For this review, take the finished solid that the model builds, in its own axes (mm). Round coordinates to 2 decimals unless told otherwise and drop trailing zeros. Loops run counter-clockwise (first coordinate to the right, second up) from the corner with the lowest first, then second, coordinate; pieces in that order, holes last.
1) Take a section at B-B (x = 16). State the section outline as (y, z) points.
2) Wall thickness on L1, parallel to Z at x = 0, y = -279.5; L2, parallel to X at y = -57, z = 16; L3, parallel to X at y = -152, z = -17: over which ranges is each line inside the solid? List them lowest first.
3) Insertion check: pin 1 (1 mm diameter, centred on y = -84.5, z = -2.5, fed in from -X); pin 2 (10 mm diameter, centred on x = 0, y = -194, fed in from -Z) (3 decimals); pin 3 (2 mm diameter, centred on x = 3, y = -97.5, fed in from +Z). Each pin has a flat end and moves straight along its axis. Give the tip position at first contact, or say it passes through.
4) Take a section at A-A (z = 17). State the section outline as (x, y) points, then the cut area to 3 significant figures.
5) Take a section at C-C (y = -317). State the section outline as (x, z) points.
6) Take a section at D-D (x = 0). State the section outline as (y, z) points, then the cut area to 3 significant figures.
```python
from build123d import *

# Parameters (mm, degrees)
F1_DEPTH = 350


with BuildPart() as f1:
    # F0 (on Front) → F1 (new body)
    with BuildSketch(Plane.XZ):
        with BuildLine():
            Line((8, -20), (20, -20))
            Line((20, -20), (20, -8))
            ThreePointArc((20, -8), (12, 0), (20, 8))
            Line((20, 8), (20, 20))
            Line((20, 20), (8, 20))
            ThreePointArc((8, 20), (0, 12), (-8, 20))
            Line((-8, 20), (-20, 20))
            Line((-20, 20), (-20, 8))
            ThreePointArc((-20, 8), (-14.343146, 5.656854), (-12, 0))
            ThreePointArc((-12, 0), (-14.343146, -5.656854), (-20, -8))
            Line((-20, -8), (-20, -20))
            Line((-20, -20), (-8, -20))
            ThreePointArc((-8, -20), (0, -12), (8, -20))
        make_face()
    extrude(amount=F1_DEPTH)


solid = f1.part
```
Response:
1. outline: (-350, -20) - (0, -20) - (0, -6.93) - (-350, -6.93) - close; (-350, 6.93) - (0, 6.93) - (0, 20) - (-350, 20) - close
2. L1: z = -12 to 12
2. L2: x = -20 to -6.93, 6.93 to 20
2. L3: x = -20 to -7.42, 7.42 to 20
3. pin 1: stops at x = -12.58
3. pin 2: stops at z = -13.755
3. pin 3: stops at z = 13.07
4. outline: (-20, -350) - (-7.42, -350) - (-7.42, 0) - (-20, 0) - close; (7.42, -350) - (20, -350) - (20, 0) - (7.42, 0) - close
4. area: 8,810 mm2
5. outline: (-20, -20) - (-8, -20) arc R8 cw to (8, -20) - (20, -20) - (20, -8) arc R8 cw to (20, 8) - (20, 20) - (8, 20) arc R8 cw to (-8, 20) - (-20, 20) - (-20, 8) arc R8 cw to (-12, 0) arc R8 cw to (-20, -8) - close
6. outline: (-350, -12) - (0, -12) - (0, 12) - (-350, 12) - close
6. area: 8,400 mm2
